The model under review builds one solid part; all positions refer to its coordinate system, in mm. A direction names the side the tool comes from. Give positions to 0.01 mm unless a question says otherwise; leave off trailing zeros. Order: outer loops, then holes, each group sorted by start corner. A loop starts at its lowest first (then second) coordinate and runs counter-clockwise, first axis right, second up. Notation, with made-up numbers: (43.5, -24) - (67.5, -24) arc R33 ccw to (67.5, 11) - close; hole circle Ø10 at (1, 9). An arc over 180 degrees is marked (long way). Use CSV: the item, a comma, the result in double quotes. Start each with the question number.
```python
from build123d import *

# Parameters (mm, degrees)
EXTRUDE_1_DEPTH = 25
FILLET_2_R      = 10
FILLET_3_R      = 10
FILLET_4_R      = 10
FILLET_6_R      = 5


with BuildPart() as part:
    # 草圖1 → 填料-伸長1 (new body)
    with BuildSketch(Plane.XY):
        with BuildLine():
            Line((-55.29380505, 11.975806452), (-55.29380505, -28.024193548))
            Line((-55.29380505, -28.024193548), (12.70619495, -28.024193548))
            Line((12.70619495, -28.024193548), (12.70619495, 2.647849462))
            Line((12.70619495, 2.647849462), (92.70619495, 2.647849462))
            Line((92.70619495, 2.647849462), (92.70619495, 8.647849462))
            Line((92.70619495, 8.647849462), (17.70619495, 8.647849462))
            ThreePointArc((17.70619495, 8.647849462), (14.170661044, 10.112315556), (12.70619495, 13.647849462))
            Line((12.70619495, 13.647849462), (12.70619495, 21.647849462))
            ThreePointArc((12.70619495, 21.647849462), (14.170661044, 25.183383368), (17.70619495, 26.647849462))
            Line((17.70619495, 26.647849462), (92.70619495, 26.647849462))
            Line((92.70619495, 26.647849462), (92.70619495, 32.647849462))
            Line((92.70619495, 32.647849462), (2.70619495, 32.647849462))
            Line((2.70619495, 32.647849462), (2.70619495, -18.024193548))
            Line((2.70619495, -18.024193548), (-47.29380505, -18.024193548))
            Line((-47.29380505, -18.024193548), (-47.29380505, 11.975806452))
            Line((-47.29380505, 11.975806452), (-55.29380505, 11.975806452))
        make_face()
    extrude(amount=EXTRUDE_1_DEPTH)

    # 圓角2
    fillet_2_edges = [part.edges().sort_by_distance(p)[0] for p in [
        (-55.29380505, -8.024193548, 0),
    ]]
    fillet(fillet_2_edges, radius=FILLET_2_R)

    # 圓角3
    fillet_3_edges = [part.edges().sort_by_distance(p)[0] for p in [
        (-55.29380505, -8.024193548, 25),
    ]]
    fillet(fillet_3_edges, radius=FILLET_3_R)

    # 圓角4
    fillet_4_edges = [part.edges().sort_by_distance(p)[0] for p in [
        (2.70619495, 7.311827957, 0),
        (2.70619495, 7.311827957, 25),
    ]]
    fillet(fillet_4_edges, radius=FILLET_4_R - 0.0001)  # a hair under: the kernel refuses the full size

    # 圓角6
    fillet_6_edges = [part.edges().sort_by_distance(p)[0] for p in [
        (-16.29385505, -18.024193548, 0),
        (-16.29385505, -18.024193548, 25),
        (-46.29889467, -18.024193548, 0.05063847),
        (-46.29889467, -18.024193548, 24.94936153),
    ]]
    fillet(fillet_6_edges, radius=FILLET_6_R)


solid = part.part
```
1. Tool access review of faces 1 (the face through (-50, 11.976, 12)), 2 (the face through (55, 26.648, 12)), 3 (the face through (52, 2.648, 12)), 4 (the face through (-16.7, -19.45, 1.504)), 5 (the face through (2.706, 8, 12)): name each direction out of +Z, -Z, +X, -X, +Y, -Y from which nothing blocks a thin tool from reaching the whole face with its end or side.
2. Mouldability with a two-part tool opening along X and no side actions: class faces 6 (the face through (92.706, 30, 12)), 7 (the face through (5.713, 4.422, 22.148)), 8 (the face through (34, 7, 25)) as pulls with the +X half, pulls with the -X half, needs draft (parallel to the pull), parting line crosses it, or undercut.
3. To check wall thickness, follow L1, parallel to Y at x = 35, z = 8; L2, parallel to X at y = -11.5, z = 11; L3, parallel to X at y = 6, z = 3.75. State the ranges of each line that lie inside material, in increasing order. Write a range as [from, to].
4. Consider section B-B (x = 70). Give the boundary of the cut face in (y, z).
5. Consider section D-D (x = -16). Give the boundary of the cut face in (y, z).
6. Clearance check with flat-ended pins moving along their axes: pin 1 (10 mm diameter, centred on x = 37.5, z = 6.5, fed in from -Y); pin 2 (7.5 mm diameter, centred on x = -14.5, z = 11, fed in from +Y); pin 3 (4 mm diameter, centred on y = 16.5, z = 16, fed in from +X). State where each tip first meets the part, or that it passes through.
Answers follow:
1,face 1,"+Z, -Z, -X, +Y"
1,face 2,"+Z, -Z, +X"
1,face 3,"+Z, -Z, +X, -Y"
1,face 4,"-Z, +Y"
1,face 5,"+Z, -Z, +Y"
2,face 6,"pulls with the +X half"
2,face 7,"undercut"
2,face 8,"needs draft"
3,L1,"y = [2.65, 8.65], [26.65, 32.65]"
3,L2,"x = [-55.29, -47.29], [2.71, 12.71]"
3,L3,"x = [-53.1, -47.29], [4.9, 92.71]"
4,outline,"(2.65, 0) - (8.65, 0) - (8.65, 25) - (2.65, 25) - close; (26.65, 0) - (32.65, 0) - (32.65, 25) - (26.65, 25) - close"
5,outline,"(-28.02, 0) - (-23.02, 0) arc R5 ccw to (-18.02, 5) - (-18.02, 20) arc R5 ccw to (-23.02, 25) - (-28.02, 25) - close"
6,pin 1,"stops at y = 2.65"
6,pin 2,"stops at y = -18.02"
6,pin 3,"stops at x = 12.71"
